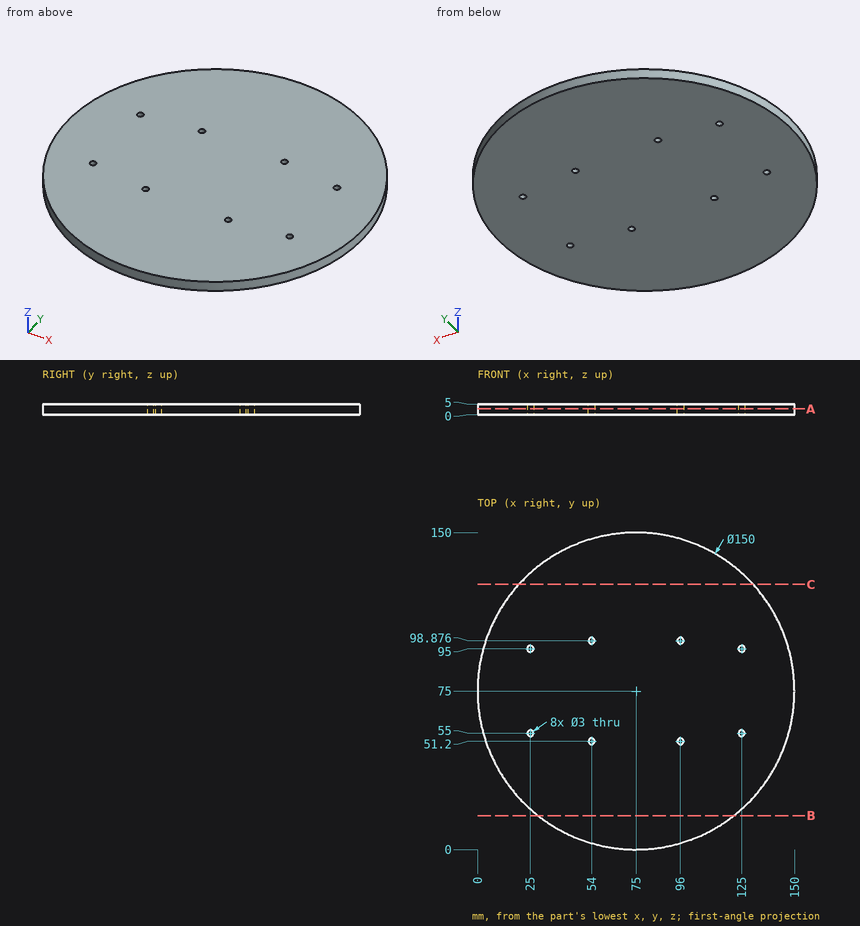
Geometry: see drawing. Coordinates: mm, zero at the bounding-box minimum. Give positions to 0.01 mm unless a question says otherwise; leave off trailing zeros. Order: outer loops, then holes, each group sorted by start corner. A loop starts at its lowest first (then second) coordinate and runs counter-clockwise, first axis right, second up. Notation, with made-up numbers: (53, 34.5) -> (109, 34.5) arc R18 ccw to (109, 39.5) -> close; hole circle Ø11 at (47, 18). An arc over 180 degrees is marked (long way). Write each question's results on one line, items separated by ' | '.
1) Line query: line 1 along Y through (x, z) = (96, 1.6); line 2 along Y through (x, z) = (25, 3.25); line 3 along X through (y, z) = (50, 1.75). Output: solid intervals per line, ascending.
Geometry says:
line 1: y = 3 to 49.7, 52.7 to 97.38, 100.38 to 147 | line 2: y = 19.1 to 53.5, 56.5 to 93.5, 96.5 to 130.9 | line 3: x = 4.29 to 53.1, 54.9 to 95.1, 96.9 to 145.71
2) Cut plane C-C (y = 125.5). Output: boundary loops of the cut face in (x, z).
Geometry says:
outline: (19.55, 0) -> (130.45, 0) -> (130.45, 5) -> (19.55, 5) -> close
3) Cut plane B-B (y = 16). Output: boundary loops of the cut face in (x, z).
Geometry says:
outline: (28.7, 0) -> (121.3, 0) -> (121.3, 5) -> (28.7, 5) -> close
4) Cut plane A-A (z = 2.65). Give the number of separate pieces and of enclosed holes in the cut face, and give its area (3 significant figures).
Geometry says:
separate pieces: 1 | enclosed holes: 8 | area: 17,600 mm²
5) First-contact query: pin 1 Ø2 at (y, z) = (103, 3.5) entering from -X; pin 2 Ø1 at (y, z) = (15.5, 2) entering from +X; pin 3 Ø1.8 at (x, y) = (54, 51.2) entering from -Z; pin 4 Ø1 at (y, z) = (33, 4) entering from +X. Flat tips, straight axial feed; report the tip coordinate or a pass-through.
Geometry says:
pin 1: stops at x = 5.03 | pin 2: stops at x = 121.3 | pin 3: passes through | pin 4: stops at x = 137.47
